Verification items for the finished model (mm, model axes). A direction names the side the tool comes from. Coordinates: 2 decimals unless noted, no trailing zeros. Loops run counter-clockwise (first coordinate to the right, second up) from the corner with the lowest first, then second, coordinate; pieces in that order, holes last. Notation, with made-up numbers: (28.25, 22) - (33.25, 22) arc R28 cw to (33.25, 41) - close; hole circle Ø5 at (54.5, 9.25). An arc over 180 degrees is marked (long way). One line per item, written item: value. Start each with the question number.
(1) Section check B-B (y = -47). Record the boundary of the cut face in (x, z), plus the area to 3 significant figures.
(2) Draft check along X on faces 4 (the face through (4.54, -44.65, 12.4)), 5 (the face through (9, -50.8, 0)), 6 (the face through (3.94, -37.87, 9.3)). Enter one of: +X half, -X half, draft (parallel to the pull), parting line (faces both ways), or undercut.
(3) Set-up check for faces 1 (the face through (4.626, -45.685, -10.15)), 2 (the face through (3.554, -40.625, 2.987)), 3 (the face through (4.54, -44.65, 9.27)): record each of +Z, -Z, +X, -X, +Y, -Y from which the full face is reachable in a straight line by a thin tool's end or side.
(4) Gauge pin test, flat ends, axial feed: P1, Ø4, axis at y = -9, z = 2.5, coming from the -X side; P2, Ø1.5, axis at x = 1.5, z = -3.5, coming from the -Y side. Record the tip position at first contact, or that the pin passes through.
(5) Thickness scan on probe 1 along Y at (x, z) = (8, -2); probe 2 along Y at (x, z) = (5.25, 6); probe 3 along Z at (x, y) = (7.25, -18.5). Record the ranges inside material, lowest first. Write a range as [from, to].
(6) Section check A-A (z = -15). Record the boundary of the cut face in (x, y), plus the area to 3 significant figures.
Autodesk Inventor part; units mm, degrees
ref_plane "Work Plane1" through (12.7, -50.8, 0) normal (0.7071, -0.7071, 0) x (0, 0, 1)
ref_plane "YZ Plane" through (0, 0, 0) normal (1, 0, 0) x (0, 1, 0)
ref_plane "XZ Plane" through (0, 0, 0) normal (0, 1, 0) x (-1, 0, 0)
sketch "Sketch1" plane through (0, 0, 0) normal (0, 0, 1) x (1, 0, 0)
  line L0 (0, 0) -> (4.4444, -50.8)
  line L1 (0, -76.2) -> (0, 12.7)
  line L2 (0, 0) -> (12.7, 0)
  line L3 (12.7, 0) -> (12.7, -50.8)
  line L4 (4.4444, -50.8) -> (12.7, -50.8)
  dimension "d0" = 5
  dimension "d1" = 12.7
  dimension "d3" = 50.8
extrude "Extrusion1" add sketch "Sketch1" along normal mid plane 38.1
ref_plane "Work Plane1" through (12.7, -50.8, 0) normal (0.7071, -0.7071, 0) x (0, 0, 1)
sketch "Sketch2" plane through (12.7, -50.8, 0) normal (0.7071, -0.7071, 0) x (0, 0, 1)
  line L0 (19.05, 0) -> (19.05, -35.921)
  line L1 (19.05, -35.921) -> (-19.05, -35.921)
  line L2 (-19.05, -35.921) -> (-19.05, 0)
  line L3 (-19.05, 0) -> (19.05, 0)
  circle A0 centre (0, -16.871) radius 11.43
  point P0 (0, -26.9408)
  dimension "d7" = 22.86
  dimension "d10" = 19.05
extrude "Extrusion2" cut sketch "Sketch2" against normal through all contours A0
sketch "Sketch3" plane through (4.4444, -50.8, -19.05) normal (-0.9962, -0.0872, 0) x (0, 0, 1)
  line L0 (0, 0) -> (0, 50.994) construction
  line L1 (0, 10.16) -> (38.1, 10.16) construction
  line L2 (38.1, 50.994) -> (38.1, 0) construction
  line L3 (0, 0) -> (38.1, 0) construction
  line L4 (13.1178, 15.24) -> (9.6187, 5.08)
  line L5 (9.6187, 5.08) -> (8.1613, 5.08)
  line L6 (8.1613, 5.08) -> (4.6622, 15.24)
  line L7 (4.6622, 15.24) -> (6.1112, 15.24)
  line L8 (6.1112, 15.24) -> (8.9271, 6.8008)
  line L9 (8.9271, 6.8008) -> (11.7429, 15.24)
  line L10 (11.7429, 15.24) -> (13.1178, 15.24)
  line L11 (17.638, 8.9085) -> (13.793, 8.9085)
  line L12 (13.793, 8.9085) -> (13.793, 10.1435)
  line L13 (13.793, 10.1435) -> (17.638, 10.1435)
  line L14 (17.638, 10.1435) -> (17.638, 8.9085)
  spline S0 degree 2 poles (25.3115, 10.16) (25.3115, 7.4265) (23.7224, 4.8659) (22.0675, 4.8659) knots 0 0 0 1 2 2 2
  spline S1 degree 2 poles (22.0675, 4.8659) (20.3879, 4.8659) (18.8153, 7.4759) (18.8153, 10.1518) knots 0 0 0 1 2 2 2
  spline S2 degree 2 poles (18.8153, 10.1518) (18.8153, 12.9017) (20.4044, 15.4458) (22.0675, 15.4458) knots 0 0 0 1 2 2 2
  spline S3 degree 2 poles (22.0675, 15.4458) (23.7389, 15.4458) (25.3115, 12.8112) (25.3115, 10.16) knots 0 0 0 1 2 2 2
  spline S4 degree 2 poles (23.566, 7.0642) (23.7636, 7.5665) (23.9283, 9.1144) (23.9283, 10.16) knots 0 0 0 1 2 2 2
  spline S5 degree 2 poles (23.9283, 10.16) (23.9283, 11.2056) (23.7636, 12.7453) (23.5578, 13.264) knots 0 0 0 1 2 2 2
  spline S6 degree 2 poles (23.5578, 13.264) (23.3519, 13.7827) (22.6356, 14.3179) (22.0675, 14.3179) knots 0 0 0 1 2 2 2
  spline S7 degree 2 poles (22.0675, 14.3179) (21.4994, 14.3179) (20.7667, 13.7827) (20.5526, 13.2475) knots 0 0 0 1 2 2 2
  spline S8 degree 2 poles (20.5526, 13.2475) (20.3468, 12.7288) (20.1986, 11.148) (20.1986, 10.1518) knots 0 0 0 1 2 2 2
  spline S9 degree 2 poles (20.1986, 10.1518) (20.1986, 9.0814) (20.3303, 7.6488) (20.5444, 7.0889) knots 0 0 0 1 2 2 2
  spline S10 degree 2 poles (20.5444, 7.0889) (20.742, 6.562) (21.4747, 5.9939) (22.0675, 5.9939) knots 0 0 0 1 2 2 2
  spline S11 degree 2 poles (22.0675, 5.9939) (22.6274, 5.9939) (23.3602, 6.5291) (23.566, 7.0642) knots 0 0 0 1 2 2 2
  line L15 (32.3675, 5.08) -> (27.411, 5.08)
  line L16 (27.411, 5.08) -> (27.411, 6.1174)
  line L17 (27.411, 6.1174) -> (29.2553, 6.1174)
  line L18 (29.2553, 6.1174) -> (29.2553, 12.9264)
  line L19 (29.2553, 12.9264) -> (27.411, 12.9264)
  line L20 (27.411, 12.9264) -> (27.411, 13.8568)
  spline S12 degree 2 poles (27.411, 13.8568) (28.4566, 13.8568) (29.4447, 14.4496) (29.5105, 15.2729) knots 0 0 0 1 2 2 2
  line L21 (29.5105, 15.2729) -> (30.5644, 15.2729)
  line L22 (30.5644, 15.2729) -> (30.5644, 6.1174)
  line L23 (30.5644, 6.1174) -> (32.3675, 6.1174)
  line L24 (32.3675, 6.1174) -> (32.3675, 5.08)
  point P0 (19.05, 50.994)
  dimension "d12" = 10.16
extrude "Extrusion3" cut sketch "Sketch3" against normal blind 1.27
equation "\"d0\" = backAngle"
equation "\"d1\" = topPartDepth"
equation "\"d3\" = partHeight"
equation "\"d4\" = partWidth"
equation "\"d7\" = pipeExteriorDiameter"
equation "\"d10\" = pipeCenter"
equation "\"d13\" = textDepth"
equation "\"topPartDepth\" = 12.7"
equation "\"backAngle\" = 5deg"
equation "\"partHeight\" = 50.8"
equation "\"partWidth\" = 38.1"
equation "\"pipeExteriorDiameter\" = 22.86"
equation "\"pipeCenter\" = 19.05"
equation "\"filletEdge\" = 1.05833"
equation "\"textDepth\" = 1.27"
properties part number "waterHeaterVent-V01"
Responses:
1. outline: (4.11, -19.05) - (12.7, -19.05) - (12.7, 19.05) - (4.11, 19.05) - close
1. area: 327 mm²
2. face 4: undercut
2. face 5: draft
2. face 6: -X half
3. face 1: -X
3. face 2: +Z, -Z, -X, -Y
3. face 3: none
4. P1: stops at x = 8.4
4. P2: stops at y = -1.18
5. probe 1: y = [-50.8, -38.16], [-6.33, 0]
5. probe 2: y = [-50.8, -33.25], [-5.73, 0]
5. probe 3: z = [-19.05, -11.23], [11.23, 19.05]
6. outline: (0, 0) - (4.44, -50.8) - (12.7, -50.8) - (12.7, 0) - close
6. area: 532 mm²
